from build123d import *

# Parameters (mm, degrees)
SKETCH1_W           = 62
SKETCH1_H           = 70
SKETCH1_W_2         = 27.5
SKETCH1_H_2         = 47.5
BOSS_EXTRUDE1_DEPTH = 1.6
CHAMFER1_SIZE       = 5
CHAMFER2_SIZE       = 6
SKETCH3_W           = 32
SKETCH3_H           = 52
BOSS_EXTRUDE2_DEPTH = 50
BOSS_EXTRUDE3_DEPTH = 5
SKETCH5_W           = 10
SKETCH5_H           = 45
CUT_EXTRUDE1_DEPTH  = 45
CHAMFER3_SIZE       = 11
CHAMFER4_SIZE       = 10
SKETCH7_R           = 2
CUT_EXTRUDE2_DEPTH  = 83.770767787
MOVE_START          = -2
MOVE_FACE1_DEPTH    = 2
SKETCH8_R           = 1.75
CUT_EXTRUDE3_DEPTH  = 74.413622714


# Read off the part's stored shape, not the designer's step: Move Face1
# Some blends are built 0.0001 mm under size
with BuildPart() as part:
    # Sketch1 → Boss-Extrude1 (new body)
    with BuildSketch(Plane.XY):
        Rectangle(SKETCH1_W, SKETCH1_H)
        Rectangle(SKETCH1_W_2, SKETCH1_H_2, mode=Mode.SUBTRACT)
    extrude(amount=BOSS_EXTRUDE1_DEPTH)

    # Chamfer1
    chamfer1_edges = [part.edges().sort_by_distance(p)[0] for p in [
        (-31, 35, 0.8),
        (31, 35, 0.8),
        (31, -35, 0.8),
        (-31, -35, 0.8),
    ]]
    chamfer(chamfer1_edges, length=CHAMFER1_SIZE)

    # Chamfer2
    chamfer2_edges = [part.edges().sort_by_distance(p)[0] for p in [
        (-13.75, -23.75, 0.8),
        (13.75, -23.75, 0.8),
    ]]
    chamfer(chamfer2_edges, length=CHAMFER2_SIZE)

    # Sketch3 → Boss-Extrude2 (add)
    with BuildSketch(Plane(origin=(0, 0, 0), x_dir=(-1, 0, 0), z_dir=(0, 0, -1))):
        with BuildLine():
            Line((-20, 27.5), (-20, -27.5))
            ThreePointArc((-20, -27.5), (-19.267766953, -29.267766953), (-17.5, -30))
            Line((-17.5, -30), (17.5, -30))
            ThreePointArc((17.5, -30), (19.267766953, -29.267766953), (20, -27.5))
            Line((20, -27.5), (20, 27.5))
            ThreePointArc((20, 27.5), (19.267766953, 29.267766953), (17.5, 30))
            Line((17.5, 30), (-17.5, 30))
            ThreePointArc((-17.5, 30), (-19.267766953, 29.267766953), (-20, 27.5))
        make_face()
        Rectangle(SKETCH3_W, SKETCH3_H, mode=Mode.SUBTRACT)
    extrude(amount=BOSS_EXTRUDE2_DEPTH)

    # Sketch4 → Boss-Extrude3 (add)
    with BuildSketch(Plane(origin=(0, 0, -50), x_dir=(-1, 0, 0), z_dir=(0, 0, -1))):
        with BuildLine():
            Line((17.5, 30), (-17.5, 30))
            ThreePointArc((-17.5, 30), (-19.267766953, 29.267766953), (-20, 27.5))
            Line((-20, 27.5), (-20, -27.5))
            ThreePointArc((-20, -27.5), (-19.267766953, -29.267766953), (-17.5, -30))
            Line((-17.5, -30), (17.5, -30))
            ThreePointArc((17.5, -30), (19.267766953, -29.267766953), (20, -27.5))
            Line((20, -27.5), (20, 27.5))
            ThreePointArc((20, 27.5), (19.267766953, 29.267766953), (17.5, 30))
        make_face()
    extrude(amount=BOSS_EXTRUDE3_DEPTH)

    # Sketch5 → Cut-Extrude1 (cut)
    with BuildSketch(Plane(origin=(0, 0, -55), x_dir=(-1, 0, 0), z_dir=(0, 0, -1))):
        with Locations((0, -7.5)):
            Rectangle(SKETCH5_W, SKETCH5_H)
    extrude(amount=-CUT_EXTRUDE1_DEPTH, mode=Mode.SUBTRACT)

    # Chamfer3
    chamfer3_edges = [part.edges().sort_by_distance(p)[0] for p in [
        (-16, 0, -50),
        (0, 26, -50),
        (16, 0, -50),
    ]]
    chamfer(chamfer3_edges, length=CHAMFER3_SIZE - 0.0001)  # a hair under: the kernel refuses the full size

    # Chamfer4
    # the kernel refuses this chamfer: 10 mm, written as the material it takes off along each edge
    with BuildSketch(Plane(origin=(-43.21682988, 30, -55), x_dir=(0, -0.9996219169112968, -0.027495876610586317), z_dir=(1, 0, 0))) as chamfer4_piece_1:
        Polygon((CHAMFER4_SIZE * 0.999621916911, -CHAMFER4_SIZE * 0.0274958766106), (-CHAMFER4_SIZE * 0.0274958766106, -CHAMFER4_SIZE * 0.999621916911), (0, 0), align=None)
    extrude(amount=86.433659759, mode=Mode.SUBTRACT)
    with BuildSketch(Plane(origin=(20, 53.21682988, -55), x_dir=(-0.9996219169112968, 0, -0.027495876610586317), z_dir=(0, -1, 0)), Plane(origin=(-20, -53.21682988, -55), x_dir=(0.9996219169112968, 0, -0.027495876610586317), z_dir=(0, 1, 0))) as chamfer4_piece_2:
        Polygon((CHAMFER4_SIZE * 0.999621916911, -CHAMFER4_SIZE * 0.0274958766106), (-CHAMFER4_SIZE * 0.0274958766106, -CHAMFER4_SIZE * 0.999621916911), (0, 0), align=None)
    extrude(amount=106.433659759, mode=Mode.SUBTRACT)

    # Sketch7 → Cut-Extrude2 (cut, through all)
    with BuildSketch(Plane(origin=(20, 0, 0), x_dir=(0, 0, -1), z_dir=(1, 0, 0))):
        with Locations(Location((4, 14.75, 0), (0, 0, 90))):
            Circle(SKETCH7_R)
        with Locations(Location((4, -12.75, 0), (0, 0, 90))):
            Circle(SKETCH7_R)
    extrude(amount=-CUT_EXTRUDE2_DEPTH, mode=Mode.SUBTRACT)

    # Move Face1 outline → Move Face1 (add)
    with BuildSketch(Plane.XY.offset(MOVE_START)):
        Polygon((-31, 30), (-31, -30), (-26, -35), (26, -35), (31, -30), (31, 30), (26, 35), (-26, 35), align=None)
        with BuildLine():
            ThreePointArc((-20, 27.5), (-19.267766953, 29.267766953), (-17.5, 30))
            Line((-17.5, 30), (17.5, 30))
            ThreePointArc((17.5, 30), (19.267766953, 29.267766953), (20, 27.5))
            Line((20, 27.5), (20, -27.5))
            ThreePointArc((20, -27.5), (19.267766953, -29.267766953), (17.5, -30))
            Line((17.5, -30), (-17.5, -30))
            ThreePointArc((-17.5, -30), (-19.267766953, -29.267766953), (-20, -27.5))
            Line((-20, -27.5), (-20, 27.5))
        make_face(mode=Mode.SUBTRACT)
    extrude(amount=MOVE_FACE1_DEPTH)

    # Sketch8 → Cut-Extrude3 (cut, through all)
    with BuildSketch(Plane.XY.offset(1.6)):
        with Locations((26, 20)):
            Circle(SKETCH8_R)
        with Locations((26, -20)):
            Circle(SKETCH8_R)
        with Locations((-26, -20)):
            Circle(SKETCH8_R)
        with Locations((-26, 20)):
            Circle(SKETCH8_R)
    extrude(amount=-CUT_EXTRUDE3_DEPTH, mode=Mode.SUBTRACT)


solid = part.part
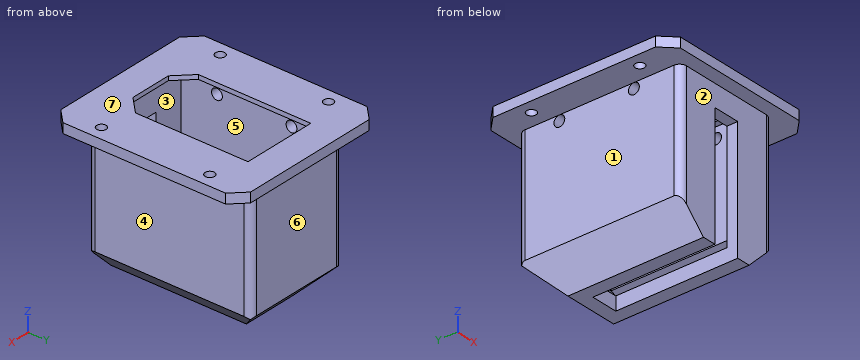
Model file for the job. Use its own axes, mm. Face numbers are marked on the shaded views. A direction names the side the tool comes from. Give positions to 0.01 mm unless a question says otherwise; leave off trailing zeros. Write each loop counter-clockwise with the first axis right and the second up, starting at its lowest first coordinate (ties: lowest second). Pieces come first, ordered by that corner, then holes. Notation, with made-up numbers: (-1.5, 71) -> (11.5, 71) arc R16 cw to (11.5, 77) -> close; hole circle Ø1 at (89, -1.5). An arc over 180 degrees is marked (long way). Write item = value, one per line.
(1) Probe line 1 along Y through (x, z) = (-17.55, -4); line 2 along Y through (x, z) = (26, 0.6); line 3 along X through (y, z) = (-5.5, -9.5). List the from-to ranges inside material, lowest first.
Determined:
line_1 = -30 to -14.75, -10.75 to 12.75, 16.75 to 30
line_2 = -35 to -21.75, -18.25 to 18.25, 21.75 to 35
line_3 = -20 to -16, 16 to 20
(2) Slice it at B-B, the plane y = -20. Give the number of separate pieces and of enclosed holes in the cut face, then the cut area to 3 significant figures.
Determined:
separate_pieces = 4
enclosed_holes = 0
area = 652 mm2
(3) Flat gauge pins, fed straight in: P1, Ø8, axis at x = -2.5, y = 17.5, coming from the +Z side; P2, Ø10, axis at x = -23.5, z = -40, coming from the -Y side; P3, Ø6.5, axis at y = 14.75, z = -4, coming from the -X side; P4, Ø9.5, axis at x = 3.5, z = -22.5, coming from the +Y side. Where does each tip first touch, or does it go through?
Determined:
P1 = -43.5
P2 = -29.79
P3 = -31
P4 = 30
(4) Tool access for the marked faces 1, 2, 3 and 4: list every direction of +Z, -Z, +X, -X, +Y, -Y with a clear straight run to the whole face (end or side of a thin tool).
Determined:
face_1 = -Z, -X, +Y, -Y
face_2 = -Z, +X, -X, -Y
face_3 = none
face_4 = -Z, +X, +Y, -Y
(5) Slice it at C-C, the plane z = -4. Give the cut face in (x, y).
Determined:
outline = (-20, -27.5) arc R2.5 ccw to (-17.5, -30) -> (17.5, -30) arc R2.5 ccw to (20, -27.5) -> (20, -14.75) -> (16, -14.75) -> (16, -26) -> (-16, -26) -> (-16, -14.75) -> (-20, -14.75) -> close; (-20, -10.75) -> (-16, -10.75) -> (-16, 12.75) -> (-20, 12.75) -> close; (-20, 16.75) -> (-16, 16.75) -> (-16, 26) -> (16, 26) -> (16, 16.75) -> (20, 16.75) -> (20, 27.5) arc R2.5 ccw to (17.5, 30) -> (-17.5, 30) arc R2.5 ccw to (-20, 27.5) -> close; (16, -10.75) -> (20, -10.75) -> (20, 12.75) -> (16, 12.75) -> close
(6) Mould opens along Y. For the marked faces 5, 6 and 7 say: released by +Y, released by -Y, zero draft, split by the parting line, or undercut.
Determined:
face_5 = undercut
face_6 = released by +Y
face_7 = zero draft
